Check sheet for the modelled part. Datum: model origin and axes. Units: mm. A direction names the side the tool comes from. Round coordinates to 2 decimals unless told otherwise and drop trailing zeros. Loops run counter-clockwise (first coordinate to the right, second up) from the corner with the lowest first, then second, coordinate; pieces in that order, holes last. Notation, with made-up numbers: (35, 48.25) -> (63, 48.25) arc R20 ccw to (63, 86.25) -> close; hole circle Ø9 at (-13.5, 24.5). An arc over 180 degrees is marked (long way). Use one line per item in the form item = value. Start each with the question number.
(1) Material ranges on probe 1 along Y at (x, z) = (0, -1.1); probe 2 along X at (y, z) = (26.5, 0.75); probe 3 along Y at (x, z) = (6.5, -1.5), recorded low to high. Write a range as [from, to].
(2) Set-up check for faces 1 (the conical face through (9.02, 5.71, 2.29)), 2 (the flat face through (-8, 4, 1)), 3 (the cylindrical face through (6.07, 12.82, -3.49)): record each of +Z, -Z, +X, -X, +Y, -Y from which the full face is reachable in a straight line by a thin tool's end or side.
(3) Go/stop test with flat-tipped pins: pin 1 (1 mm diameter, centred on y = 26, z = 1.5, fed in from -X); pin 2 (0.6 mm diameter, centred on y = 4, z = 1.5, fed in from +X); pin 3 (0.8 mm diameter, centred on x = 0, y = 28, fed in from +Z). Record where each tip stops, or that it passes through.
(4) Sectioned sample at B-B (y = 10.25). Record the cut outline in (x, z).
(5) Sectioned sample at D-D (z = -3). Record the cut outline in (x, y), and give its area (3 significant figures).
(6) Sectioned sample at C-C (x = 2). Record the cut outline in (y, z).
(7) Draft check along X on faces 4 (the flat face through (-10, 4, 1)), 5 (the cylindrical face through (10.125, 14.79, -4.298)), 6 (the flat face through (-9, 4, 2.4)), 7 (the flat face through (-8, 26, 1)). Enter one of: released by +X, released by -X, zero draft, split by the parting line, or undercut.
(8) Sectioned sample at A-A (z = 1). Record the cut outline in (x, y), and give its area (3 significant figures).
from build123d import *

# Parameters (mm, degrees)
F1_W      = 22
F1_H      = 30
F2_DEPTH  = 8
F4_DEPTH  = 30.001
F6_DEPTH  = 2.4
F7_SIZE   = 0.4
F9_DEPTH  = 26
F10_R     = 0.5
F11_DEPTH = 4


with BuildPart() as f2:
    # F1 (on Top) → F2 (new body)
    with BuildSketch(Plane.XY):
        with Locations((0, 15)):
            Rectangle(F1_W, F1_H)
    extrude(amount=-F2_DEPTH)

    # F3 (on face) → F4 (cut, through all)
    with BuildSketch(Plane.XZ):
        with BuildLine():
            ThreePointArc((-7.549834, -8), (-10.100697, -4.356135), (-11, 0))
            Line((-11, 0), (-11, -8))
            Line((-11, -8), (-7.549834, -8))
        make_face()
        with BuildLine():
            Line((11, -8), (11, 0))
            ThreePointArc((11, 0), (10.100697, -4.356135), (7.549834, -8))
            Line((7.549834, -8), (11, -8))
        make_face()
    extrude(amount=-F4_DEPTH, mode=Mode.SUBTRACT)

    # F5 (on face) → F6 (join)
    with BuildSketch(Plane.XY):
        with BuildLine():
            ThreePointArc((-8, 5), (-9, 6), (-10, 5))
            Line((-10, 5), (-10, 3))
            ThreePointArc((-10, 3), (-9, 2), (-8, 3))
            Line((-8, 3), (-8, 5))
        make_face()
        with BuildLine():
            ThreePointArc((10, 5), (9, 6), (8, 5))
            Line((8, 5), (8, 3))
            ThreePointArc((8, 3), (9, 2), (10, 3))
            Line((10, 3), (10, 5))
        make_face()
        with BuildLine():
            ThreePointArc((-8, 27), (-9, 28), (-10, 27))
            Line((-10, 27), (-10, 25))
            ThreePointArc((-10, 25), (-9, 24), (-8, 25))
            Line((-8, 25), (-8, 27))
        make_face()
        with BuildLine():
            ThreePointArc((10, 27), (9, 28), (8, 27))
            Line((8, 27), (8, 25))
            ThreePointArc((8, 25), (9, 24), (10, 25))
            Line((10, 25), (10, 27))
        make_face()
    extrude(amount=F6_DEPTH)

    # F7
    f7_edges = [f2.edges().sort_by_distance(p)[0] for p in [
        (-9, 6, 2.4),
        (-10, 4, 2.4),
        (-9, 2, 2.4),
        (-8, 4, 2.4),
        (9, 6, 2.4),
        (8, 4, 2.4),
        (9, 2, 2.4),
        (10, 4, 2.4),
        (-9, 28, 2.4),
        (-10, 26, 2.4),
        (-9, 24, 2.4),
        (-8, 26, 2.4),
        (9, 28, 2.4),
        (8, 26, 2.4),
        (9, 24, 2.4),
        (10, 26, 2.4),
    ]]
    chamfer(f7_edges, length=F7_SIZE)

    # F8 (on face) → F9 (cut)
    with BuildSketch(Plane.XZ):
        with BuildLine():
            Line((7, 0), (-7, 0))
            ThreePointArc((-7, 0), (-6.092572, -3.44682), (-3.605551, -6))
            Line((-3.605551, -6), (3.605551, -6))
            ThreePointArc((3.605551, -6), (6.092572, -3.44682), (7, 0))
        make_face()
    extrude(amount=-F9_DEPTH, mode=Mode.SUBTRACT)

    # F10 (on face) → F11 (cut)
    with BuildSketch(Plane.XY):
        with Locations((0, 28)):
            Circle(F10_R)
    extrude(amount=-F11_DEPTH, mode=Mode.SUBTRACT)


solid = f2.part
Checks:
q1.probe_1 = [26, 27.5], [28.5, 30]
q1.probe_2 = [-10, -8], [8, 10]
q1.probe_3 = [26, 30]
q2.face_1 = +Z
q2.face_2 = +Z, +Y, -Y
q2.face_3 = +Z, -Y
q3.pin_1 = -10
q3.pin_2 = 10
q3.pin_3 = -4
q4.outline = (-11, 0) arc R11 ccw to (-7.55, -8) -> (7.55, -8) arc R11 ccw to (11, 0) -> (7, 0) arc R7 cw to (3.61, -6) -> (-3.61, -6) arc R7 cw to (-7, 0) -> close
q5.outline = (-10.58, 0) -> (-6.32, 0) -> (-6.32, 26) -> (6.32, 26) -> (6.32, 0) -> (10.58, 0) -> (10.58, 30) -> (-10.58, 30) -> close; hole circle Ø1 at (0, 28)
q5.area = 305 mm2
q6.outline = (0, -8) -> (30, -8) -> (30, 0) -> (26, 0) -> (26, -6) -> (0, -6) -> close
q7.face_4 = released by -X
q7.face_5 = released by +X
q7.face_6 = zero draft
q7.face_7 = undercut
q8.outline = (-10, 3) arc R1 ccw to (-8, 3) -> (-8, 5) arc R1 ccw to (-10, 5) -> close; (-10, 25) arc R1 ccw to (-8, 25) -> (-8, 27) arc R1 ccw to (-10, 27) -> close; (8, 3) arc R1 ccw to (10, 3) -> (10, 5) arc R1 ccw to (8, 5) -> close; (8, 25) arc R1 ccw to (10, 25) -> (10, 27) arc R1 ccw to (8, 27) -> close
q8.area = 28.6 mm2
